Read the model definition and answer for the solid it produces. Units are mm, in the model's axes. Give positions to 0.01 mm unless a question says otherwise; leave off trailing zeros. Order: outer loops, then holes, each group sorted by start corner. A loop starts at its lowest first (then second) coordinate and runs counter-clockwise, first axis right, second up. Notation, with made-up numbers: (57, 72.5) -> (101, 72.5) arc R13 ccw to (101, 85.5) -> close; hole circle Ø3 at (87.5, -40). An arc over 180 degrees is marked (long way). Use one line per item in the form item = value.
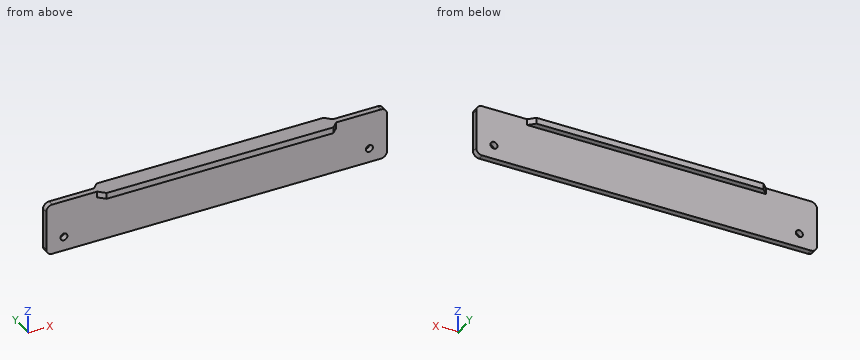
```python
from build123d import *

# Parameters (mm, degrees)
SKETCH1_W           = 170
SKETCH1_H           = 25.4
BOSS_EXTRUDE1_DEPTH = 3
FILLET1_R           = 3
SKETCH2_R           = 1.75
CUT_EXTRUDE1_DEPTH  = 3
SKETCH3_W           = 119.2
SKETCH3_H           = 9
BOSS_EXTRUDE2_DEPTH = 3
CHAMFER1_SIZE       = 3


with BuildPart() as part:
    # Sketch1 → Boss-Extrude1 (new body)
    with BuildSketch(Plane(origin=(0, 0, 0), x_dir=(1, 0, 0), z_dir=(0, 1, 0))):
        with Locations((10.053763441, 8.016845878)):
            Rectangle(SKETCH1_W, SKETCH1_H)
    extrude(amount=BOSS_EXTRUDE1_DEPTH)

    # Fillet1
    fillet1_edges = [part.edges().sort_by_distance(p)[0] for p in [
        (-74.946236559, 1.5, -20.716845878),
        (95.053763441, 1.5, -20.716845878),
        (95.053763441, 1.5, 4.683154122),
        (-74.946236559, 1.5, 4.683154122),
    ]]
    fillet(fillet1_edges, radius=FILLET1_R)

    # Sketch2 → Cut-Extrude1 (cut)
    with BuildSketch(Plane(origin=(0, 3, 0), x_dir=(1, 0, 0), z_dir=(0, 1, 0))):
        with Locations(Location((86.253763441, 13.716845878, 0), (0, 0, 270))):
            Circle(SKETCH2_R)
        with Locations(Location((-66.146236559, 13.716845878, 0), (0, 0, 270))):
            Circle(SKETCH2_R)
    extrude(amount=-CUT_EXTRUDE1_DEPTH, mode=Mode.SUBTRACT)

    # Sketch3 → Boss-Extrude2 (add)
    with BuildSketch(Plane.XY.offset(4.683154122)):
        with Locations((10.053763441, 1.5)):
            Rectangle(SKETCH3_W, SKETCH3_H)
    extrude(amount=-BOSS_EXTRUDE2_DEPTH)

    # Chamfer1
    chamfer1_edges = [part.edges().sort_by_distance(p)[0] for p in [
        (-49.546236559, -3, 3.183154122),
        (69.653763441, -3, 3.183154122),
        (69.653763441, 6, 3.183154122),
        (-49.546236559, 6, 3.183154122),
    ]]
    chamfer(chamfer1_edges, length=CHAMFER1_SIZE - 0.0001)  # a hair under: the kernel refuses the full size


solid = part.part
```
Item 1: Given pin 1 Ø1 at (x, z) = (-6.5, -14.5) entering from +Y; pin 2 Ø1.5 at (x, y) = (22.5, 5) entering from -Z; pin 3 Ø5.5 at (x, z) = (-66.15, -13.72) entering from -Y; pin 4 Ø1 at (y, z) = (5, -18) entering from -X, each flat-ended and moving along its own axis, determine where each tip first touches the part or whether it passes through.
Checks:
pin_1 = 3
pin_2 = 1.68
pin_3 = 0
pin_4 = through
Item 2: The part is cut by section A-A on x = 58.5. Give the vertices of the cut face in (y, z), and give its area (3 significant figures).
Checks:
outline = (-3, 1.68) -> (0, 1.68) -> (0, -20.72) -> (3, -20.72) -> (3, 1.68) -> (6, 1.68) -> (6, 4.68) -> (-3, 4.68) -> close
area = 94.2 mm²
Item 3: The part is cut by section B-B on z = -3. Give the vertices of the cut face in (x, y).
Checks:
outline = (-74.95, 0) -> (95.05, 0) -> (95.05, 3) -> (-74.95, 3) -> close
Item 4: Straight lines are drawn through the part: L1, parallel to Z at x = 41, y = -0.25; L2, parallel to Y at x = 56, z = -15; L3, parallel to Y at x = -49, z = 3.75. For each, find the intervals that lie inside material, in ascending order. Write a range as from..to.
Checks:
L1 = 1.68..4.68
L2 = 0..3
L3 = -0.55..3.55
Item 5: The part is cut by section C-C on x = 75.5. Give the vertices of the cut face in (y, z), and give its area (3 significant figures).
Checks:
outline = (0, -20.72) -> (3, -20.72) -> (3, 4.68) -> (0, 4.68) -> close
area = 76.2 mm²
